from build123d import *

# Parameters (mm, degrees)
SKETCH1_W           = 86
SKETCH1_H           = 86
SKETCH1_R           = 19
BOSS_EXTRUDE1_DEPTH = 12
CUT_EXTRUDE1_REACH  = 14
SKETCH2_R           = 3.3
SKETCH4_R           = 36.5
CUT_EXTRUDE2_DEPTH  = 1.8
SKETCH6_W           = 8.07061303
SKETCH6_H           = 12
CUT_EXTRUDE3_DEPTH  = 13


with BuildPart() as part:
    # Sketch1 → Boss-Extrude1 (new body)
    with BuildSketch(Plane(origin=(0, 0, 0), x_dir=(1, 0, 0), z_dir=(0, 1, 0))):
        Rectangle(SKETCH1_W, SKETCH1_H)
        Circle(SKETCH1_R, mode=Mode.SUBTRACT)
    extrude(amount=BOSS_EXTRUDE1_DEPTH)

    # Sketch2 → Cut-Extrude1 (cut, up to next)
    with BuildSketch(Plane(origin=(0, 12, 0), x_dir=(1, 0, 0), z_dir=(0, 1, 0)), mode=Mode.PRIVATE) as cut_extrude1_sk1:
        with Locations((-34.507589913, -34.373280458)):
            Circle(SKETCH2_R)
    cut_extrude1_tool1 = extrude(cut_extrude1_sk1.sketch, amount=-CUT_EXTRUDE1_REACH, mode=Mode.PRIVATE) & part.part
    add(cut_extrude1_tool1.solids().sort_by_distance((-34.50759, 12, 34.37328))[0], mode=Mode.SUBTRACT)
    # Sketch2 → Cut-Extrude1 (cut, up to next)
    with BuildSketch(Plane(origin=(0, 12, 0), x_dir=(1, 0, 0), z_dir=(0, 1, 0)), mode=Mode.PRIVATE) as cut_extrude1_sk2:
        with Locations((-34.507589913, 35.126719542)):
            Circle(SKETCH2_R)
    cut_extrude1_tool2 = extrude(cut_extrude1_sk2.sketch, amount=-CUT_EXTRUDE1_REACH, mode=Mode.PRIVATE) & part.part
    add(cut_extrude1_tool2.solids().sort_by_distance((-34.50759, 12, -35.12672))[0], mode=Mode.SUBTRACT)
    # Sketch2 → Cut-Extrude1 (cut, up to next)
    with BuildSketch(Plane(origin=(0, 12, 0), x_dir=(1, 0, 0), z_dir=(0, 1, 0)), mode=Mode.PRIVATE) as cut_extrude1_sk3:
        with Locations((34.992410087, -34.373280458)):
            Circle(SKETCH2_R)
    cut_extrude1_tool3 = extrude(cut_extrude1_sk3.sketch, amount=-CUT_EXTRUDE1_REACH, mode=Mode.PRIVATE) & part.part
    add(cut_extrude1_tool3.solids().sort_by_distance((34.99241, 12, 34.37328))[0], mode=Mode.SUBTRACT)
    # Sketch2 → Cut-Extrude1 (cut, up to next)
    with BuildSketch(Plane(origin=(0, 12, 0), x_dir=(1, 0, 0), z_dir=(0, 1, 0)), mode=Mode.PRIVATE) as cut_extrude1_sk4:
        with Locations((34.992410087, 35.126719542)):
            Circle(SKETCH2_R)
    cut_extrude1_tool4 = extrude(cut_extrude1_sk4.sketch, amount=-CUT_EXTRUDE1_REACH, mode=Mode.PRIVATE) & part.part
    add(cut_extrude1_tool4.solids().sort_by_distance((34.99241, 12, -35.12672))[0], mode=Mode.SUBTRACT)

    # Sketch4 → Cut-Extrude2 (cut)
    with BuildSketch(Plane(origin=(0, 12, 0), x_dir=(1, 0, 0), z_dir=(0, 1, 0))):
        with Locations((0.242410087, 0.376719542)):
            Circle(SKETCH4_R)
    extrude(amount=-CUT_EXTRUDE2_DEPTH, mode=Mode.SUBTRACT)

    # Sketch6 → Cut-Extrude3 (cut, through all)
    with BuildSketch(Plane(origin=(0, 12, 0), x_dir=(1, 0, 0), z_dir=(0, 1, 0))):
        with Locations((-41.851719536, 0)):
            Rectangle(SKETCH6_W, SKETCH6_H)
    extrude(amount=-CUT_EXTRUDE3_DEPTH, mode=Mode.SUBTRACT)


solid = part.part
Verification items for the finished model (mm, model axes). A direction names the side the tool comes from. Coordinates: 2 decimals unless noted, no trailing zeros. Order: outer loops, then holes, each group sorted by start corner. A loop starts at its lowest first (then second) coordinate and runs counter-clockwise, first axis right, second up. Notation, with made-up numbers: (4.25, 42) -> (8.25, 42) arc R31 cw to (8.25, 76) -> close; hole circle Ø11 at (87.25, -16). An arc over 180 degrees is marked (long way). Use CSV: the item, a comma, the result in double quotes. Start each with the question number.
Q1. Tool access check on faces 4 (the flat face through (16, 10.2, 15)), 5 (the flat face through (-37.816, 6, 0)), 6 (the flat face through (-43, 6, 25)). Record the directions out of +Z, -Z, +X, -X, +Y, -Y that give a thin tool (end or side, any length) a straight path to the whole face; none if there is none.
Q2. Section check B-B, the plane x = -8.5. Record the cut outline in (y, z).
Q3. Section check C-C, the plane y = 1. Record the cut outline in (x, z).
Q4. Section check D-D, the plane z = -22. Record the cut outline in (x, y).
Q5. Depth check by flat-ended pin: P1, Ø1.5, axis at y = 10.5, z = 0, coming from the -X side; P2, Ø4, axis at x = 34.99, z = 34.37, coming from the +Y side. Enter the tip coordinate at first touch or a pass-through.
Q6. Thickness scan on line 1 along Z through (x, y) = (-32, 1.5); line 2 along X through (y, z) = (3.25, 35.5); line 3 along X through (y, z) = (6, 0). Record the ranges inside material, lowest first.
Q7. Draft check along X on faces 1 (the cylindrical face through (17.085, 11.113, 32.005)), 2 (the flat face through (-1, 6, -43)), 3 (the flat face through (-43, 6, -24)). Enter one of: +X half, -X half, draft (parallel to the pull), parting line (faces both ways), or undercut.
Q8. Section check A-A, the plane z = 4.5. Record the cut outline in (x, y).
Returned:
1,face 4,"+Y"
1,face 5,"-X, +Y, -Y"
1,face 6,"+Z, -Z, -X, +Y, -Y"
2,outline,"(0, -43) -> (12, -43) -> (12, -35.81) -> (10.2, -35.81) -> (10.2, -16.99) -> (0, -16.99) -> close; (0, 16.99) -> (10.2, 16.99) -> (10.2, 35.06) -> (12, 35.06) -> (12, 43) -> (0, 43) -> close"
3,outline,"(-43, -43) -> (43, -43) -> (43, 43) -> (-43, 43) -> (-43, 6) -> (-37.82, 6) -> (-37.82, -6) -> (-43, -6) -> close; hole circle Ø6.6 at (-34.51, -35.13); hole circle Ø6.6 at (-34.51, 34.37); hole circle Ø38 at (0, 0); hole circle Ø6.6 at (34.99, -35.13); hole circle Ø6.6 at (34.99, 34.37)"
4,outline,"(-43, 0) -> (43, 0) -> (43, 12) -> (29.65, 12) -> (29.65, 10.2) -> (-29.16, 10.2) -> (-29.16, 12) -> (-43, 12) -> close"
5,P1,"stops at x = -37.82"
5,P2,"passes through"
6,line 1,"z = -43 to -37.27, -32.98 to 32.23, 36.52 to 43"
6,line 2,"x = -43 to -37.61, -31.41 to 31.89, 38.09 to 43"
6,line 3,"x = -37.82 to -19, 19 to 43"
7,face 1,"undercut"
7,face 2,"draft"
7,face 3,"-X half"
8,outline,"(-37.82, 0) -> (-18.46, 0) -> (-18.46, 10.2) -> (-35.93, 10.2) -> (-35.93, 12) -> (-37.82, 12) -> close; (18.46, 0) -> (43, 0) -> (43, 12) -> (36.42, 12) -> (36.42, 10.2) -> (18.46, 10.2) -> close"
